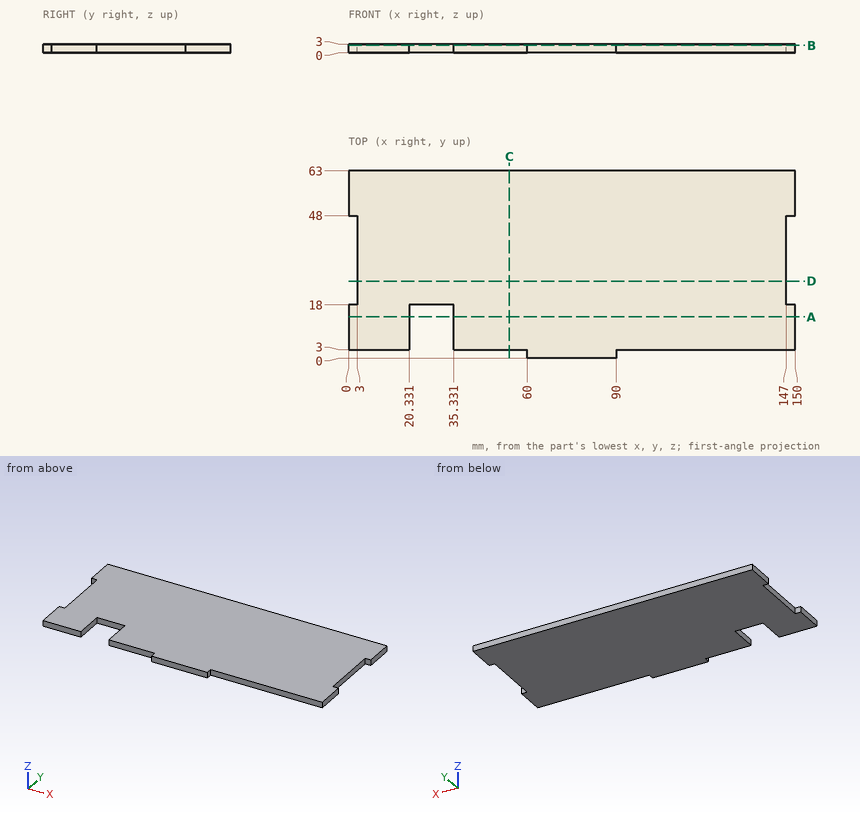
Geometry: see drawing. Coordinates: mm, zero at the bounding-box minimum. Give positions to 0.01 mm unless a question says otherwise; leave off trailing zeros. Write each loop counter-clockwise with the first axis right and the second up, starting at its lowest first coordinate (ties: lowest second). Pieces come first, ordered by that corner, then holes. Notation, with made-up numbers: (85, -25) - (105, -25) arc R12 cw to (105, -20) - close; hole circle Ø3 at (28.5, 56.25). An arc over 180 degrees is marked (long way). Return JSON: item names as keys, results as strings. Group by question number.
1) First-contact query: P1, Ø0.9, axis at x = 108, z = 2, coming from the -Y side; P2, Ø1.5, axis at x = 28, z = 1.5, coming from the -Y side; P3, Ø0.9, axis at y = 36.5, z = 1.5, coming from the -X side. Flat tips, straight axial feed; report the tip coordinate or a pass-through.
2) Section D-D on y = 26. Return the cut outline in (x, z).
3) Section B-B on z = 2.55. Return the cut outline in (x, y), plus the area to 4 significant figures.
4) Line query: line 1 (X direction, y = 11, z = 2); line 2 (X direction, y = 24, z = 0.7); line 3 (Y direction, x = 53.5, z = 0.75). Output: solid intervals per line, ascending.
5) Section A-A on y = 14. Return the cut outline in (x, z).
6) Section C-C on x = 54. Return the cut outline in (y, z), plus the area to 3 significant figures.
Filled in:
{
 "1": {"P1": "stops at y = 3", "P2": "stops at y = 18", "P3": "stops at x = 3"},
 "2": {"outline": "(3, 0) - (147, 0) - (147, 3) - (3, 3) - close"},
 "3": {"outline": "(0, 3) - (20.33, 3) - (20.33, 18) - (35.33, 18) - (35.33, 3) - (60, 3) - (60, 0) - (90, 0) - (90, 3) - (150, 3) - (150, 18) - (147, 18) - (147, 48) - (150, 48) - (150, 63) - (0, 63) - (0, 48) - (3, 48) - (3, 18) - (0, 18) - close", "area": "8,685 mm^2"},
 "4": {"line 1": "x = 0 to 20.33, 35.33 to 150", "line 2": "x = 3 to 147", "line 3": "y = 3 to 63"},
 "5": {"outline": "(0, 0) - (20.33, 0) - (20.33, 3) - (0, 3) - close; (35.33, 0) - (150, 0) - (150, 3) - (35.33, 3) - close"},
 "6": {"outline": "(3, 0) - (63, 0) - (63, 3) - (3, 3) - close", "area": "180 mm^2"}
}
